Verification items for the finished model (mm, model axes). A direction names the side the tool comes from. Round coordinates to 2 decimals unless told otherwise and drop trailing zeros. Write each loop counter-clockwise with the first axis right and the second up, starting at its lowest first coordinate (ties: lowest second). Pieces come first, ordered by that corner, then holes. Notation, with made-up numbers: (-15.5, 11.25) -> (-8.5, 11.25) arc R16 ccw to (-8.5, 41.25) -> close; hole circle Ø7 at (-24.5, -10.5). An arc over 180 degrees is marked (long way). Use CSV: the item, a comma, the result in double quotes.
```python
from build123d import *

# Parameters (mm, degrees)
BASESKETCH_W             = 16
BASESKETCH_H             = 300
BASE_DEPTH               = 46
SHAPESKETCH_OUTSIDE_W    = 362.786
SHAPESKETCH_OUTSIDE_H    = 108.786
SHAPE_DEPTH              = 17
SUPPORTR_DEPTH           = 3
SUPPORTL_START           = -16
SUPPORTL_DEPTH           = 3
CONNECTIONCENTERSKETCH_W = 10.1
CONNECTIONCENTERSKETCH_H = 3.1
CONNECTIONCENTER_DEPTH   = 10
WEIGHTL_DEPTH            = 57.736422329
WEIGHTR_DEPTH            = 57.736422329
CONNECTIONEND_DEPTH      = 7
CONNECTIONEND_DEPTH_BACK = 50
SHORTNERSKETCH_W         = 17.734474479
SHORTNERSKETCH_H         = 84.123631353
SHORTNERSKETCH_W_2       = 27.514011897
SHORTNERSKETCH_H_2       = 94.21863772
CUT_EXTRUDE1_DEPTH       = 17


with BuildPart() as part:
    # BaseSketch → Base (new body)
    with BuildSketch(Plane(origin=(0, 0, 0), x_dir=(1, 0, 0), z_dir=(0, 1, 0))):
        Rectangle(BASESKETCH_W, BASESKETCH_H)
    extrude(amount=BASE_DEPTH)

    # ShapeSketch outside → Shape (cut, through all)
    with BuildSketch(Plane(origin=(8, 0, 0), x_dir=(0, 0, -1), z_dir=(1, 0, 0))):
        with Locations((0, 23)):
            Rectangle(SHAPESKETCH_OUTSIDE_W, SHAPESKETCH_OUTSIDE_H)
        Polygon((-23, 3), (23, 3), (120, 43), (150, 43), (150, 46), (120, 46), (23, 6), (-23, 6), (-120, 46), (-150, 46), (-150, 43), (-120, 43), align=None, mode=Mode.SUBTRACT)
    extrude(amount=-SHAPE_DEPTH, mode=Mode.SUBTRACT)

    # SupportSketch → SupportR (add)
    with BuildSketch(Plane.ZY.offset(8)):
        Polygon((-150, 52), (-150, 43), (-120, 43), (-23, -3), (23, -3), (120, 43), (150, 43), (150, 52), (120, 52), (23, 6), (-23, 6), (-120, 52), align=None)
    extrude(amount=-SUPPORTR_DEPTH)

    # SupportSketch<3> → SupportL (add)
    with BuildSketch(Plane.ZY.offset(8).offset(SUPPORTL_START)):
        Polygon((-150, 52), (-150, 43), (-120, 43), (-23, -3), (23, -3), (120, 43), (150, 43), (150, 52), (120, 52), (23, 6), (-23, 6), (-120, 52), align=None)
    extrude(amount=SUPPORTL_DEPTH)

    # ConnectionCenterSketch → ConnectionCenter (cut, through all)
    with BuildSketch(Plane(origin=(0, 6, 0), x_dir=(1, 0, 0), z_dir=(0, 1, 0))):
        with Locations((0, -18.5)):
            Rectangle(CONNECTIONCENTERSKETCH_W, CONNECTIONCENTERSKETCH_H)
        with Locations((0, 18.5)):
            Rectangle(CONNECTIONCENTERSKETCH_W, CONNECTIONCENTERSKETCH_H)
    extrude(amount=-CONNECTIONCENTER_DEPTH, mode=Mode.SUBTRACT)

    # WeightLSketch → WeightL (cut, through all)
    with BuildSketch(Plane(origin=(0, -2.97810882, 1.228086111), x_dir=(1, 0, 0), z_dir=(0, 0.924480592, -0.38122911))):
        Polygon((-5, -124.474210145), (-5, -112.474210145), (5, -118.700707453), align=None)
        Polygon((5, -114.700707453), (5, -102.700707453), (-5, -108.927204761), align=None)
        Polygon((-5, -104.927204761), (-5, -92.927204761), (5, -99.153702069), align=None)
        Polygon((5, -95.153702069), (5, -83.153702069), (-5, -89.380199377), align=None)
        Polygon((5, -79.606696685), (-5, -85.380199377), (-5, -73.380199377), align=None)
        Polygon((5, -75.606696685), (5, -63.606696685), (-5, -69.833193994), align=None)
        Polygon((-5, -46.28618861), (-5, -34.28618861), (5, -40.512685918), align=None)
        Polygon((-5, -65.833193994), (-5, -53.833193994), (5, -60.059691302), align=None)
        Polygon((5, -56.059691302), (5, -44.059691302), (-5, -50.28618861), align=None)
        Polygon((5, -36.512685918), (5, -24.512685918), (-5, -30.739183226), align=None)
    extrude(amount=-WEIGHTL_DEPTH, mode=Mode.SUBTRACT)

    # WeightRSketch → WeightR (cut, through all)
    with BuildSketch(Plane(origin=(0, -2.97810882, -1.228086111), x_dir=(1, 0, 0), z_dir=(0, 0.924480592, 0.38122911))):
        Polygon((5, 125.474210145), (5, 113.474210145), (-5, 119.700707453), align=None)
        Polygon((-5, 115.700707453), (-5, 103.700707453), (5, 109.474210145), align=None)
        Polygon((5, 105.474210145), (5, 93.474210145), (-5, 99.700707453), align=None)
        Polygon((-5, 95.700707453), (-5, 83.700707453), (5, 89.927204761), align=None)
        Polygon((5, 85.927204761), (5, 73.927204761), (-5, 79.700707453), align=None)
        Polygon((-5, 75.700707453), (-5, 63.700707453), (5, 69.927204761), align=None)
        Polygon((5, 65.927204761), (5, 53.927204761), (-5, 60.153702069), align=None)
        Polygon((-5, 56.153702069), (-5, 44.153702069), (5, 50.380199377), align=None)
        Polygon((5, 46.380199377), (5, 34.380199377), (-5, 40.606696685), align=None)
        Polygon((-5, 36.606696685), (-5, 24.606696685), (5, 30.833193994), align=None)
    extrude(amount=-WEIGHTR_DEPTH, mode=Mode.SUBTRACT)

    # ConnectionEndSketch → ConnectionEnd (cut, two sides)
    with BuildSketch(Plane(origin=(0, 46, 0), x_dir=(1, 0, 0), z_dir=(0, 1, 0))) as connectionend_sk:
        with BuildLine():
            Line((2, 134), (2, 125))
            ThreePointArc((2, 125), (0, 123), (-2, 125))
            Line((-2, 125), (-2, 134))
            ThreePointArc((-2, 134), (0, 136), (2, 134))
        make_face()
        with BuildLine():
            Line((-2, -134), (-2, -125))
            ThreePointArc((-2, -125), (0, -123), (2, -125))
            Line((2, -125), (2, -134))
            ThreePointArc((2, -134), (0, -136), (-2, -134))
        make_face()
    extrude(amount=CONNECTIONEND_DEPTH, mode=Mode.SUBTRACT)
    extrude(connectionend_sk.sketch, amount=-CONNECTIONEND_DEPTH_BACK, mode=Mode.SUBTRACT)

    # ShortnerSketch → Cut-Extrude1 (cut, through all)
    with BuildSketch(Plane.ZY.offset(8)):
        with Locations((-148.86723724, 42.061815677)):
            Rectangle(SHORTNERSKETCH_W, SHORTNERSKETCH_H)
        with Locations((153.757005949, 47.10931886)):
            Rectangle(SHORTNERSKETCH_W_2, SHORTNERSKETCH_H_2)
    extrude(amount=-CUT_EXTRUDE1_DEPTH, mode=Mode.SUBTRACT)


solid = part.part
```
Q1. Material ranges on L1, parallel to X at y = 0, z = 23.5; L2, parallel to Y at x = -4.5, z = 5; L3, parallel to Z at x = 4.5, y = 25.5, recorded low to high.
Filled in:
L1,"-8 to -5, 5 to 8"
L2,"3 to 6"
L3,"70.96 to 75.26, 75.91 to 77.56"
Q2. Access from +Z, -Z, +X, -X, +Y, -Y to the whole of each face (thin tool, end or side, straight path). Record for faces 1 (the flat face through (4, 43, 130)), 2 (the flat face through (0.07, 37.873, 107.567)), 3 (the flat face through (-1.041, 7.047, 25.538)).
Filled in:
face 1,"+Z, +X, -X, -Y"
face 2,"+Z, -Y"
face 3,"+Y"
Q3. Mould release check, pull along X, two halves, no side actions. Record for faces 4 (the flat face through (-6.521, 20.322, -72.179)), 5 (the flat face through (0, 5, -16.95)): released by +X, released by -X, zero draft, split by the parting line, or undercut.
Filled in:
face 4,"zero draft"
face 5,"undercut"
Q4. Go/stop test with flat-tipped pins: P1, Ø4.5, axis at x = 0, y = 0.5, coming from the -Z side; P2, Ø2, axis at x = 3, y = 31, coming from the +Z side; P3, Ø3, axis at x = 2, z = -126.5, coming from the +Y side; P4, Ø2.5, axis at x = -1.5, z = 22, coming from the -Y side. Record where each tip stops, or that it passes through.
Filled in:
P1,"through"
P2,"z = 93.06"
P3,"y = 46"
P4,"y = 3"
Q5. Section check A-A (z = -9.5). Record the cut outline in (x, y).
Filled in:
outline,"(-8, -3) -> (-5, -3) -> (-5, 3) -> (5, 3) -> (5, -3) -> (8, -3) -> (8, 6) -> (-8, 6) -> close"
